from build123d import *

# Parameters (mm, degrees)
SKETCH1_W           = 26.4
SKETCH1_H           = 34.3
SKETCH1_R           = 1.575
BOSS_EXTRUDE1_DEPTH = 1.5
SKETCH3_W           = 12.5
SKETCH3_H           = 2.5
BOSS_EXTRUDE2_DEPTH = 2.5
SWEEP3_START        = 7.89
SWEEP3_DEPTH        = 0.62
LPATTERN1_COUNT     = 5
LPATTERN1_PITCH     = 2.5
CUT_EXTRUDE1_DEPTH  = 2.5
CHAMFER1_SIZE       = 0.2


# Read off the part's stored shape, not the designer's step: Sweep3
with BuildPart() as part:
    # Sketch1 → Boss-Extrude1 (new body)
    with BuildSketch(Plane(origin=(0, 0, 0), x_dir=(1, 0, 0), z_dir=(0, 1, 0))):
        with Locations((13.2, 17.15)):
            Rectangle(SKETCH1_W, SKETCH1_H)
        with Locations(Location((3.375, 31.225, 0), (0, 0, 270))):
            Circle(SKETCH1_R, mode=Mode.SUBTRACT)
        with Locations(Location((23.025, 31.225, 0), (0, 0, 270))):
            Circle(SKETCH1_R, mode=Mode.SUBTRACT)
        with Locations(Location((23.025, 5.375, 0), (0, 0, 270))):
            Circle(SKETCH1_R, mode=Mode.SUBTRACT)
        with Locations(Location((3.375, 5.375, 0), (0, 0, 270))):
            Circle(SKETCH1_R, mode=Mode.SUBTRACT)
    extrude(amount=BOSS_EXTRUDE1_DEPTH)

    # Sketch3 → Boss-Extrude2 (add)
    with BuildSketch(Plane(origin=(0, 1.5, 0), x_dir=(1, 0, 0), z_dir=(0, 1, 0))):
        with Locations((13.2, 2.75)):
            Rectangle(SKETCH3_W, SKETCH3_H)
    extrude(amount=BOSS_EXTRUDE2_DEPTH)

    # Sweep3 outline → Sweep3 (add)
    with BuildSketch(Plane.YZ.offset(SWEEP3_START)):
        with BuildLine():
            Line((4, -2.44), (4, -3.06))
            add(Edge.make_bspline(
                [(4, -3.06), (4.241666667, -3.06), (4.483333333, -3.06), (4.845833333, -3.06), (4.966666667, -3.06), (5.147916667, -3.06), (5.208333333, -3.06), (5.298958333, -3.06), (5.329166667, -3.06), (5.389583333, -3.06), (5.401070283, -3.060067636), (5.503005944, -3.05992673), (5.595306319, -3.045739717), (5.730552262, -2.99013888), (5.793507671, -2.948451924), (5.898451924, -2.843507671), (5.94013888, -2.780552262), (5.995739717, -2.645306319), (6.00992673, -2.553005944), (6.010045188, -2.467309888), (6.01, -2.459635417), (6.01, -2.419270833), (6.01, -2.399088542), (6.01, -2.338541667), (6.01, -2.298177083), (6.01, -2.177083333), (6.01, -2.096354167), (6.01, -1.854166667), (6.01, -1.692708333), (6.01, -1.208333333), (6.01, -0.885416667), (6.01, 0.083333333), (6.01, 0.729166667), (6.01, 2.666666667), (6.01, 3.958333333), (6.01, 5.25)],
                knots=[0, 0, 0, 0, 0.075578312, 0.075578312, 0.113367467, 0.113367467, 0.132262045, 0.132262045, 0.141709334, 0.141709334, 0.151156623, 0.151156623, 0.161390945, 0.161390945, 0.171625267, 0.171625267, 0.181859589, 0.181859589, 0.192093911, 0.192093911, 0.198405677, 0.198405677, 0.204717443, 0.204717443, 0.217340976, 0.217340976, 0.242588041, 0.242588041, 0.293082172, 0.293082172, 0.394070433, 0.394070433, 0.596046955, 0.596046955, 1, 1, 1, 1], degree=3))
            Line((6.01, 5.25), (5.39, 5.25))
            Line((5.39, 5.25), (5.389999999, -2.440036459))
            Line((5.389999999, -2.440036459), (4, -2.44))
        make_face()
    sweep3 = extrude(amount=SWEEP3_DEPTH)

    # LPattern1: Sweep3 ×5
    with Locations(*[(i * LPATTERN1_PITCH, 0, 0) for i in range(1, LPATTERN1_COUNT)]):
        add(sweep3)

    # Sketch13 → Cut-Extrude1 (cut)
    with BuildSketch(Plane(origin=(0, 4, 0), x_dir=(1, 0, 0), z_dir=(0, 1, 0))):
        Polygon((11.95, 1.7), (11.75, 1.5), (12.15, 1.5), align=None)
        Polygon((16.75, 4), (16.95, 3.8), (17.15, 4), align=None)
        Polygon((14.45, 3.8), (14.65, 4), (14.25, 4), align=None)
        Polygon((9.45, 3.8), (9.65, 4), (9.25, 4), align=None)
        Polygon((9.25, 1.5), (9.45, 1.7), (9.65, 1.5), align=None)
        Polygon((14.45, 1.7), (14.65, 1.5), (14.25, 1.5), align=None)
        Polygon((16.75, 1.5), (17.15, 1.5), (16.95, 1.7), align=None)
        Polygon((12.15, 4), (11.75, 4), (11.95, 3.8), align=None)
    extrude(amount=-CUT_EXTRUDE1_DEPTH, mode=Mode.SUBTRACT)

    # Chamfer1
    chamfer1_edges = [part.edges().sort_by_distance(p)[0] for p in [
        (6.95, 2.75, -4),
        (6.95, 2.75, -1.5),
        (19.45, 2.75, -1.5),
        (19.45, 2.75, -4),
    ]]
    chamfer(chamfer1_edges, length=CHAMFER1_SIZE)


solid = part.part
Geometry: final body of the model. Coordinates: model frame, mm. A direction names the side the tool comes from. Round coordinates to 2 decimals unless told otherwise and drop trailing zeros. Order: outer loops, then holes, each group sorted by start corner. A loop starts at its lowest first (then second) coordinate and runs counter-clockwise, first axis right, second up.
Q1. Mould query, pull axis X, two halves, no side actions, for faces 4 (the face through (7.89, 5.7, 0.2)), 5 (the face through (11, 3, -1.5)), 6 (the face through (26.4, 1, -17)), 7 (the face through (16.01, 5.7, 0.2)). Classes: released by +X, released by -X, zero draft, split by the parting line, or undercut.
Result sheet:
face 4: released by -X
face 5: zero draft
face 6: released by +X
face 7: undercut
Q2. Pin query (flat end, axial travel): pin 1 (1.1 mm diameter, centred on x = 8.5, y = 3.5, fed in from +Z); pin 2 (1.6 mm diameter, centred on y = 5, z = -0.5, fed in from -X); pin 3 (0.6 mm diameter, centred on y = 5, z = 3, fed in from -X); pin 4 (0.5 mm diameter, centred on x = 10.5, y = 4.5, fed in from +Z). Return the tip coordinate at first contact, or that it passes through.
Result sheet:
pin 1: stops at z = -1.5
pin 2: stops at x = 7.89
pin 3: passes through
pin 4: stops at z = -2.44
Q3. Material intervals for probe 1 along Z at (x, y) = (11, 1.25); probe 2 along Z at (x, y) = (11.75, 3.75); probe 3 along Y at (x, z) = (8, -31), sorted ascending.
Result sheet:
probe 1: z = -34.3 to 0
probe 2: z = -4 to -1.5
probe 3: y = 0 to 1.5
Q4. Section C-C, the plane x = 4. Output: boundary loops of the cut face in (y, z), and give its area (3 significant figures).
Result sheet:
outline: (0, -34.3) - (1.5, -34.3) - (1.5, -32.67) - (0, -32.67) - close; (0, -29.78) - (1.5, -29.78) - (1.5, -6.82) - (0, -6.82) - close; (0, -3.93) - (1.5, -3.93) - (1.5, 0) - (0, 0) - close
area: 42.8 mm2
Q5. Access query for faces 1 (the face through (16, 3, -1.5)), 2 (the face through (10.39, 5.7, 0.2)), 3 (the face through (13, 3, -4)). Directions: +Z, -Z, +X, -X, +Y, -Y. A direction counts if a zero-diameter tool reaches every point of the face in a straight line with its end or side. Return the directions, or none.
Result sheet:
face 1: +Z, +X, -X
face 2: +Z, -Z, +Y
face 3: -Z, +X, -X, +Y
Q6. Section D-D, the plane y = 5. Give the number of separate pieces and of enclosed holes in the cut face, and give its area (3 significant figures).
Result sheet:
separate pieces: 5
enclosed holes: 0
area: 1.92 mm2
Q7. Section A-A, the plane z = -6. Output: boundary loops of the cut face in (x, y).
Result sheet:
outline: (0, 0) - (1.93, 0) - (1.93, 1.5) - (0, 1.5) - close; (4.82, 0) - (21.58, 0) - (21.58, 1.5) - (4.82, 1.5) - close; (24.47, 0) - (26.4, 0) - (26.4, 1.5) - (24.47, 1.5) - close
